```python
from build123d import *

# Parameters (mm, degrees)
SKETCH1_R           = 11.5
SKETCH1_R_2         = 1.8
BOSS_EXTRUDE1_DEPTH = 5
EXTRUDE_THIN1_START = 5
EXTRUDE_THIN1_DEPTH = 5
FILLET1_R           = 1
FILLET2_R           = 1.5


with BuildPart() as part:
    # Sketch1 → Boss-Extrude1 (new body)
    with BuildSketch(Plane.XY):
        Circle(SKETCH1_R)
        with Locations((0, 8)):
            Circle(SKETCH1_R_2, mode=Mode.SUBTRACT)
        with Locations((8, 0)):
            Circle(SKETCH1_R_2, mode=Mode.SUBTRACT)
        with Locations((0, -8)):
            Circle(SKETCH1_R_2, mode=Mode.SUBTRACT)
        with Locations((-8, 0)):
            Circle(SKETCH1_R_2, mode=Mode.SUBTRACT)
        with BuildLine():
            Line((1.557401682, 1.61), (-1.557401682, 1.61))
            ThreePointArc((-1.557401682, 1.61), (0, -2.24), (1.557401682, 1.61))
        make_face(mode=Mode.SUBTRACT)
    extrude(amount=BOSS_EXTRUDE1_DEPTH)

    # Sketch1<4> → Extrude-Thin1 (add)
    with BuildSketch(Plane.XY.offset(EXTRUDE_THIN1_START)):
        with BuildLine():
            Line((2.223848016, 3.61), (-2.223848016, 3.61))
            ThreePointArc((-2.223848016, 3.61), (0, -4.24), (2.223848016, 3.61))
        make_face()
        with BuildLine():
            Line((1.557401682, 1.61), (-1.557401682, 1.61))
            ThreePointArc((-1.557401682, 1.61), (0, -2.24), (1.557401682, 1.61))
        make_face(mode=Mode.SUBTRACT)
    extrude(amount=EXTRUDE_THIN1_DEPTH)

    # Fillet1
    fillet1_edges = [part.edges().sort_by_distance(p)[0] for p in [
        (0, 3.61, 5),
        (0, -4.24, 5),
    ]]
    fillet(fillet1_edges, radius=FILLET1_R)

    # Fillet2
    fillet2_edges = [part.edges().sort_by_distance(p)[0] for p in [
        (0, 1.61, 10),
        (0, -2.24, 10),
    ]]
    fillet(fillet2_edges, radius=FILLET2_R)


solid = part.part
```
The listing builds one solid part. Answer for the finished solid, in the listing's coordinates (mm). A direction names the side the tool comes from. Give positions to 0.01 mm unless a question says otherwise; leave off trailing zeros. Loops run counter-clockwise (first coordinate to the right, second up) from the corner with the lowest first, then second, coordinate; pieces in that order, holes last. Notation, with made-up numbers: (-9, 30) - (-5, 30) arc R17 ccw to (-5, 44) - close; hole circle Ø9 at (-4, 80.5). An arc over 180 degrees is marked (long way). Answer as CSV lines item,"result". Start each with the question number.
Item 1: A cutting plane is placed at C-C on x = -9.5. Determine the outline of the cut face in (y, z).
Item 2: A cutting plane is placed at B-B on y = -6.75. Determine the outline of the cut face in (x, z), then the cut area to 3 significant figures.
Item 3: A cutting plane is placed at A-A on x = 0. Determine the outline of the cut face in (y, z), then the cut area to 3 significant figures.
Item 4: The mould has two halves that part along Y. Classify faces 1 (the face through (-0.07, -2.24, 4.19)), 2 (the face through (0, 3.61, 8)), 3 (the face through (-0.154, -4.237, 7.972)), 4 (the face through (5, -2.4, 5)): +Y half, -Y half, draft (parallel to the pull), parting line (faces both ways), or undercut.
Item 5: A cutting plane is placed at D-D on z = 6.75. Determine the outline of the cut face in (x, y).
Item 6: For faces 5 (the face through (-0.2, -2.4, 0)), 6 (the face through (0, 1.61, 4)), 7 (the face through (-0.03, 2.06, 9.57)), determine the directions among +Z, -Z, +X, -X, +Y, -Y from which every point of the face is accessible in a straight line to the end or side of a thin tool.
Item 7: Each of these flat-tipped pins is pushed along its axis until it touches: pin 1 (2 mm diameter, centred on x = 8, y = 0, fed in from +Z); pin 2 (2 mm diameter, centred on y = 2.5, z = 9, fed in from -X); pin 3 (1.5 mm diameter, centred on y = 6, z = 4.5, fed in from +X); pin 4 (2 mm diameter, centred on x = 1, z = 9, fed in from +Y). Where does it stop, or does it pass through?
Item 8: Find the intervals of material crossed by line 1 (Y direction, x = 0, z = 3); line 2 (Y direction, x = 0.75, z = 2.5); line 3 (Z direction, x = -5.5, y = 2), in increasing order. Write a range as from..to.
Found:
1,outline,"(-6.48, 0) - (-0.99, 0) - (-0.99, 5) - (-6.48, 5) - close; (0.99, 0) - (6.48, 0) - (6.48, 5) - (0.99, 5) - close"
2,outline,"(-9.31, 0) - (-1.3, 0) - (-1.3, 5) - (-9.31, 5) - close; (1.3, 0) - (9.31, 0) - (9.31, 5) - (1.3, 5) - close"
2,area,"80.2 mm^2"
3,outline,"(-11.5, 0) - (-9.8, 0) - (-9.8, 5) - (-11.5, 5) - close; (-6.2, 0) - (-2.24, 0) - (-2.24, 8.5) arc R1.5 ccw to (-3.74, 10) - (-4.24, 10) - (-4.24, 6) arc R1 cw to (-5.24, 5) - (-6.2, 5) - close; (1.61, 0) - (6.2, 0) - (6.2, 5) - (4.61, 5) arc R1 cw to (3.61, 6) - (3.61, 10) - (3.11, 10) arc R1.5 ccw to (1.61, 8.5) - close; (9.8, 0) - (11.5, 0) - (11.5, 5) - (9.8, 5) - close"
3,area,"79.2 mm^2"
4,face 1,"undercut"
4,face 2,"+Y half"
4,face 3,"parting line"
4,face 4,"draft"
5,outline,"(-2.22, 3.61) arc R4.24 ccw (long way) to (2.22, 3.61) - close; hole (-1.56, 1.61) arc R2.24 ccw (long way) to (1.56, 1.61) - close"
6,face 5,"-Z, +X, -X, +Y, -Y"
6,face 6,"+Z, -Z"
6,face 7,"+Z"
7,pin 1,"passes through"
7,pin 2,"stops at x = -3.97"
7,pin 3,"stops at x = 10.23"
7,pin 4,"stops at y = 3.61"
8,line 1,"y = -11.5..-9.8, -6.2..-2.24, 1.61..6.2, 9.8..11.5"
8,line 2,"y = -11.48..-9.64, -6.36..-2.11, 1.61..6.36, 9.64..11.48"
8,line 3,"z = 0..5"
